Read the model definition and answer for the solid it produces. Units are mm, in the model's axes. A direction names the side the tool comes from. Coordinates: 2 decimals unless noted, no trailing zeros. Write each loop counter-clockwise with the first axis right and the second up, starting at its lowest first coordinate (ties: lowest second). Pieces come first, ordered by that corner, then holes.
from build123d import *

# Parameters (mm, degrees)
BOSS_EXTRUDE1_DEPTH     = 12.7
SKETCH7_W               = 13.75
SKETCH7_H               = 0.65
CUT_EXTRUDE2_DEPTH      = 4
SKETCH7_4_R             = 1.6
BOSS_EXTRUDE2_DEPTH     = 1.4
CUT_EXTRUDE3_DEPTH      = 4.5
SKETCH7_6_R             = 1.85
CUT_EXTRUDE4_DEPTH      = 2.4
CUT_EXTRUDE4_DEPTH_BACK = 10.7
CUT_EXTRUDE5_DEPTH      = 3
SKETCH12_W              = 1.5
SKETCH12_H              = 22.5
CUT_EXTRUDE6_DEPTH      = 3
SKETCH14_W              = 2.2
SKETCH14_H              = 4
BOSS_EXTRUDE3_DEPTH     = 1
FILLET5_R               = 1.5
FILLET6_R               = 0.25


with BuildPart() as part:
    # Sketch1 → Boss-Extrude1 (new body)
    with BuildSketch(Plane(origin=(0, 0, 0), x_dir=(1, 0, 0), z_dir=(0, 1, 0))):
        Polygon((-28.77817965, 16.29419618), (-24.27817965, 16.29419618), (-24.27817965, 25.04419618), (-22.07817965, 25.04419618), (-22.07817965, 16.29419618), (-19.07817965, 16.29419618), (-19.07817965, 2.54419618), (-28.77817965, 2.54419618), align=None)
    extrude(amount=BOSS_EXTRUDE1_DEPTH)

    # Sketch7 → Cut-Extrude2 (cut)
    with BuildSketch(Plane.ZY.offset(28.77817965)):
        with Locations((-9.41919618, 11.875)):
            Rectangle(SKETCH7_W, SKETCH7_H)
    extrude(amount=-CUT_EXTRUDE2_DEPTH, mode=Mode.SUBTRACT)

    # Sketch7<4> → Boss-Extrude2 (add)
    with BuildSketch(Plane.ZY.offset(28.77817965)):
        with Locations((-13.04419618, 9.2)):
            Circle(SKETCH7_4_R)
    extrude(amount=BOSS_EXTRUDE2_DEPTH)

    # Sketch7<5> → Cut-Extrude3 (cut)
    with BuildSketch(Plane.ZY.offset(28.77817965)):
        Polygon((-2.54419618, 0.097302003), (-16.29419618, 9.2), (-16.29419618, 0), (-2.54419618, 0), align=None)
    extrude(amount=-CUT_EXTRUDE3_DEPTH, mode=Mode.SUBTRACT)

    # Sketch7<6> → Cut-Extrude4 (cut, two sides)
    with BuildSketch(Plane.ZY.offset(28.77817965)) as cut_extrude4_sk:
        with Locations((-19.91919618, 9.2)):
            Circle(SKETCH7_6_R)
    extrude(amount=CUT_EXTRUDE4_DEPTH, mode=Mode.SUBTRACT)
    extrude(cut_extrude4_sk.sketch, amount=-CUT_EXTRUDE4_DEPTH_BACK, mode=Mode.SUBTRACT)

    # Sketch10 → Cut-Extrude5 (cut)
    with BuildSketch(Plane(origin=(-22.07817965, 0, 0), x_dir=(0, 0, -1), z_dir=(1, 0, 0))):
        Polygon((16.29419618, 9.2), (16.29419618, 0), (2.54419618, 0), (2.54419618, 0.097302003), align=None)
    extrude(amount=CUT_EXTRUDE5_DEPTH, mode=Mode.SUBTRACT)

    # Sketch12 → Cut-Extrude6 (cut)
    with BuildSketch(Plane.XZ):
        with Locations((-23.17817965, -13.79419618)):
            Rectangle(SKETCH12_W, SKETCH12_H)
    extrude(amount=-CUT_EXTRUDE6_DEPTH, mode=Mode.SUBTRACT)

    # Sketch14 → Boss-Extrude3 (add)
    with BuildSketch(Plane(origin=(0, 0, 0), x_dir=(-1, 0, 0), z_dir=(0, -1, 0))):
        with Locations((23.17817965, 4.54419618)):
            Rectangle(SKETCH14_W, SKETCH14_H)
    extrude(amount=-BOSS_EXTRUDE3_DEPTH)

    # Mirror3: part across plane


with BuildPart() as part_1:
    add(part.part)
    add(part.part.mirror(Plane(origin=(-19.07817965, 12.7, -2.54419618), x_dir=(1, 0, 0), z_dir=(0, 0, -1))))

    # Fillet5
    fillet5_edges = [part_1.edges().sort_by_distance(p)[0] for p in [
        (-19.07817965, 12.7, -2.54419618),
        (-19.07817965, 10.95, -16.29419618),
        (-26.52817965, 12.7, 11.20580382),
        (-19.07817965, 10.95, 11.20580382),
        (-19.07817965, 4.648651002, 4.33080382),
        (-20.57817965, 12.7, 11.20580382),
        (-20.57817965, 9.2, 11.20580382),
        (-23.17817965, 12.7, 19.95580382),
        (-24.10317965, 0, 19.95580382),
        (-22.25317965, 0, 19.95580382),
        (-26.52817965, 9.2, 11.20580382),
        (-20.57817965, 0.097302003, -2.54419618),
        (-20.57817965, 12.7, -16.29419618),
        (-23.17817965, 12.7, -25.04419618),
        (-26.52817965, 12.7, -16.29419618),
        (-26.52817965, 9.2, -16.29419618),
        (-19.07817965, 4.648651002, -9.41919618),
        (-20.57817965, 9.2, -16.29419618),
        (-24.10317965, 0, -25.04419618),
        (-22.25317965, 0, -25.04419618),
    ]]
    fillet(fillet5_edges, radius=FILLET5_R)

    # Fillet6
    fillet6_edges = [part_1.edges().sort_by_distance(p)[0] for p in [
        (-23.92817965, 0, -15.04419618),
        (-23.92817965, 1, -2.54419618),
        (-23.92817965, 0.5, -6.54419618),
        (-23.17817965, 1, -6.54419618),
        (-22.42817965, 0.5, -6.54419618),
        (-22.42817965, 1, -2.54419618),
        (-23.17817965, 0, -6.54419618),
        (-23.17817965, 3, 19.95580382),
        (-22.42817965, 2.25, 19.95580382),
        (-23.92817965, 0, 9.95580382),
        (-23.92817965, 2.25, 19.95580382),
        (-22.42817965, 0.5, 1.45580382),
        (-23.92817965, 0.5, 1.45580382),
        (-23.17817965, 0, 1.45580382),
        (-23.17817965, 1, 1.45580382),
        (-22.42817965, 0, -15.04419618),
        (-22.42817965, 0, 9.95580382),
        (-22.42817965, 0.439339828, -24.604856352),
        (-22.42817965, 0.439339828, 19.516463992),
        (-23.92817965, 0.439339828, -24.604856352),
        (-23.92817965, 0.439339828, 19.516463992),
        (-22.42817965, 3, -2.54419618),
        (-23.17817965, 3, -25.04419618),
        (-22.42817965, 2.25, -25.04419618),
        (-23.92817965, 3, -2.54419618),
        (-23.92817965, 2.25, -25.04419618),
    ]]
    fillet(fillet6_edges, radius=FILLET6_R)


solid = part_1.part
Item 1: For faces 1 (the cylindrical face through (-21.318, 12.272, 10.755)), 2 (the flat face through (-26.56, 4.366, 3.903)), 3 (the cylindrical face through (-21.318, 0.396, -2.556)), 4 (the flat face through (-26.56, 4.366, -8.992)), determine the directions among +Z, -Z, +X, -X, +Y, -Y from which every point of the face is accessible in a straight line to the end or side of a thin tool.
Item 2: Given pin 1 (2 mm diameter, centred on x = -22.5, z = -5.5, fed in from -Y); pin 2 (0.8 mm diameter, centred on y = 1.5, z = -1.5, fed in from -X); pin 3 (3 mm diameter, centred on x = -28.5, z = -1, fed in from -Y); pin 4 (3 mm diameter, centred on x = -26.5, z = -4.5, fed in from -Y), each flat-ended and moving along its own axis, determine where each tip first touches the part or whether it passes through.
Item 3: The part is cut by section C-C (y = 9.2). State how many separate pieces and enclosed holes the cut face has, and give its area (3 significant figures).
Item 4: Find the intervals of material crossed by probe 1 along X at (y, z) = (1.5, -5); probe 2 along X at (y, z) = (5.5, -20.5); probe 3 along Y at (x, z) = (-23.25, -22), in increasing order.
Item 5: The part is cut by section A-A (x = -25.75). Give the vertices of the cut face in (y, z), and give its area (3 significant figures).
Item 6: The part is cut by section B-B (x = -21.5). Give the vertices of the cut face in (y, z).
Answer:
1. face 1: +Z, +X, +Y
1. face 2: +Z, -X, -Y
1. face 3: +X, -Y
1. face 4: -Z, -X, -Y
2. pin 1: stops at y = 0
2. pin 2: stops at x = -28.78
2. pin 3: stops at y = 0.13
2. pin 4: stops at y = 0.4
3. separate pieces: 3
3. enclosed holes: 0
3. area: 293 mm2
4. probe 1: x = -24.28 to -23.93, -22.43 to -22.08
4. probe 2: x = -24.28 to -22.08
4. probe 3: y = 3 to 12.7
5. outline: (0.1, -2.54) - (8.76, -15.62) arc R1.5 ccw to (10.01, -16.29) - (11.2, -16.29) arc R1.5 ccw to (11.55, -16.25) - (11.55, 11.16) arc R1.5 ccw to (11.2, 11.21) - (10.01, 11.21) arc R1.5 ccw to (8.76, 10.53) - close; (12.2, -15.91) arc R1.5 ccw to (12.7, -14.79) - (12.7, 9.71) arc R1.5 ccw to (12.2, 10.82) - close
5. area: 203 mm2
6. outline: (0.65, -3.37) - (8.76, -15.62) arc R1.5 ccw to (10.01, -16.29) - (11.2, -16.29) arc R1.5 ccw to (12.7, -14.79) - (12.7, 9.71) arc R1.5 ccw to (11.2, 11.21) - (10.01, 11.21) arc R1.5 ccw to (8.76, 10.53) - (0.65, -1.72) arc R1.5 ccw to start
